The listing builds one solid part. Answer for the finished solid, in the listing's coordinates (mm). A direction names the side the tool comes from. Give positions to 0.01 mm unless a question says otherwise; leave off trailing zeros. Write each loop counter-clockwise with the first axis right and the second up, starting at its lowest first coordinate (ties: lowest second). Pieces come first, ordered by that corner, then holes. Notation, with made-up numbers: (8, 57) -> (60, 57) arc R22 ccw to (60, 71) -> close; hole circle Ø10 at (7.25, -38.5). An arc over 180 degrees is marked (long way). One line per question, with ' | ' between items.
from build123d import *

# Parameters (mm, degrees)
BOSS_EXTRUDE1_DEPTH = 60
FILLET1_R           = 20
FILLET2_R           = 50
SKETCH2_W           = 848.571428571
SKETCH2_H           = 25
CUT_EXTRUDE1_DEPTH  = 1199.832765652
FILLET3_R           = 15
BOSS_EXTRUDE2_DEPTH = 60
CHAMFER1_START      = 59.982172039
CHAMFER1_OUTLINE_W  = 43
CHAMFER1_OUTLINE_H  = 75
CHAMFER1_DEPTH      = 21.017827961
CHAMFER2_START      = 59.982172039
CHAMFER2_OUTLINE_W  = 43
CHAMFER2_OUTLINE_H  = 75
CHAMFER2_DEPTH      = 21.017827961
FILLET4_R           = 5


with BuildPart() as part:
    # Sketch1 → Boss-Extrude1 (new, symmetric)
    with BuildSketch(Plane.XY):
        Polygon((0, 0), (0, -630), (-980, -630), (-980, -645), (-380, -680), (40, -680), (40, 0), align=None)
    extrude(amount=BOSS_EXTRUDE1_DEPTH, both=True)

    # Fillet1
    fillet1_edges = [part.edges().sort_by_distance(p)[0] for p in [
        (0, -630, 0),
    ]]
    fillet(fillet1_edges, radius=FILLET1_R)

    # Fillet2
    fillet2_edges = [part.edges().sort_by_distance(p)[0] for p in [
        (40, -680, 0),
    ]]
    fillet(fillet2_edges, radius=FILLET2_R)

    # Sketch2 → Cut-Extrude1 (cut, through all)
    with BuildSketch(Plane.XY.offset(60)):
        with Locations((-384.285714286, -667.5)):
            Rectangle(SKETCH2_W, SKETCH2_H)
    extrude(amount=-CUT_EXTRUDE1_DEPTH, mode=Mode.SUBTRACT)

    # Fillet3
    fillet3_edges = [part.edges().sort_by_distance(p)[0] for p in [
        (-980, -637.5, 60),
        (-980, -637.5, -60),
    ]]
    fillet(fillet3_edges, radius=FILLET3_R)

    # Sketch4 → Boss-Extrude2 (add, symmetric)
    with BuildSketch(Plane.XY):
        Polygon((40, -45), (80, -45), (80, -112), (62, -112), (55.812506017, -95), (40, -95), align=None)
        Polygon((40, -604), (56.540446486, -604), (62, -589), (80, -589), (80, -599), (70.900744143, -624), (40, -624), align=None)
    extrude(amount=BOSS_EXTRUDE2_DEPTH, both=True)

    # Chamfer1: read off the stored shape, not the designer's step
    # Chamfer1 outline → Chamfer1 (cut)
    with BuildSketch(Plane(origin=(0, 0, 0), x_dir=(0.74035690193716, -0.281696772444383, -0.6103430069628291), z_dir=(0.6722139969935248, 0.3102526139970119, 0.6722139969935248)).offset(CHAMFER1_START)):
        with Locations((33.5, -89.5)):
            Rectangle(CHAMFER1_OUTLINE_W, CHAMFER1_OUTLINE_H)
    extrude(amount=CHAMFER1_DEPTH, mode=Mode.SUBTRACT)

    # Chamfer2: read off the stored shape, not the designer's step
    # Chamfer2 outline → Chamfer2 (cut)
    with BuildSketch(Plane(origin=(0, 0, 0), x_dir=(0.74035690193716, -0.281696772444383, 0.6103430069628291), z_dir=(0.6722139969935248, 0.3102526139970119, -0.6722139969935248)).offset(CHAMFER2_START)):
        with Locations((33.5, 89.5)):
            Rectangle(CHAMFER2_OUTLINE_W, CHAMFER2_OUTLINE_H)
    extrude(amount=CHAMFER2_DEPTH, mode=Mode.SUBTRACT)

    # Fillet4
    # the kernel refuses this fillet: 5 mm, written as the material it adds along each edge
    with BuildSketch(Plane(origin=(40, -624, -60), x_dir=(1, 0, 0), z_dir=(0, 0, 1))) as fillet4_piece_1:
        with BuildLine():
            CenterArc((FILLET4_R, -FILLET4_R), FILLET4_R, 90, 90)
            Line((0, -FILLET4_R), (0, 0))
            Line((0, 0), (FILLET4_R, 0))
        make_face()
    extrude(amount=120)
    # the kernel refuses this fillet: 5 mm, written as the material it takes off along each edge
    with BuildSketch(Plane(origin=(75, -50, 29.869584766), x_dir=(0, 0.45647233632715695, -0.8897376052342775), z_dir=(0.7504731319703868, 0.5880284369504243, 0.30168300503707374))) as fillet4_2_piece_1_section:
        Polygon((-8.486724439, -8.486724439), (8.486724439, -8.486724439), (8.486724439, 8.486724439), (-8.486724439, 8.486724439), align=None)
    fillet4_2_piece_1 = extrude(amount=8.486724439, mode=Mode.PRIVATE)
    fillet4_2_piece_1 = split(fillet4_2_piece_1, bisect_by=Plane(origin=(75, -50, 29.869584766), z_dir=(0, 0.9079593845004515, -0.41905817746174745)), keep=Keep.TOP, mode=Mode.PRIVATE)
    fillet4_2_piece_1 = split(fillet4_2_piece_1, bisect_by=Plane(origin=(75, -50, 29.869584766), z_dir=(0.7071067811865476, 0, -0.7071067811865476)), keep=Keep.TOP, mode=Mode.PRIVATE)
    fillet4_2_piece_1 = split(fillet4_2_piece_1, bisect_by=Plane(origin=(75, -50, 29.869584766), z_dir=(0, 0, 1)), keep=Keep.TOP, mode=Mode.PRIVATE)
    fillet4_2_piece_1 = split(fillet4_2_piece_1, bisect_by=Plane(origin=(80, -50, 29.869584766), z_dir=(-1, 0, 0)), keep=Keep.TOP, mode=Mode.PRIVATE)
    fillet4_2_piece_1 = split(fillet4_2_piece_1, bisect_by=Plane(origin=(78.361069985, -48.44873693, 33.230654751), z_dir=(-0.6722139969935248, -0.3102526139970119, -0.6722139969935248)), keep=Keep.TOP, mode=Mode.PRIVATE)
    fillet4_2_piece_1 = split(fillet4_2_piece_1, bisect_by=Plane(origin=(75, -45, 29.869584766), z_dir=(0, -1, 0)), keep=Keep.TOP, mode=Mode.PRIVATE)
    fillet4_2_piece_1 = fillet4_2_piece_1 - Plane(origin=(75, -50, 29.869584766), x_dir=(-0.7504731319703868, -0.5880284369504243, -0.30168300503707374), z_dir=(0, 0.45647233632715695, -0.8897376052342775)) * Sphere(FILLET4_R, mode=Mode.PRIVATE)
    add(fillet4_2_piece_1, mode=Mode.SUBTRACT)
    with BuildSketch(Plane(origin=(75, -50, -29.869584766), x_dir=(-0.6608271381079537, 0.6608271381079537, -0.3558299974427439), z_dir=(0.7504731319703868, 0.5880284369504243, -0.30168300503707374))) as fillet4_2_piece_2_section:
        Polygon((-8.486724439, -8.486724439), (8.486724439, -8.486724439), (8.486724439, 8.486724439), (-8.486724439, 8.486724439), align=None)
    fillet4_2_piece_2 = extrude(amount=8.486724439, mode=Mode.PRIVATE)
    fillet4_2_piece_2 = split(fillet4_2_piece_2, bisect_by=Plane(origin=(75, -50, -29.869584766), z_dir=(0, 0.9079593845004515, 0.41905817746174745)), keep=Keep.TOP, mode=Mode.PRIVATE)
    fillet4_2_piece_2 = split(fillet4_2_piece_2, bisect_by=Plane(origin=(75, -50, -29.869584766), z_dir=(0, 0, -1)), keep=Keep.TOP, mode=Mode.PRIVATE)
    fillet4_2_piece_2 = split(fillet4_2_piece_2, bisect_by=Plane(origin=(75, -50, -29.869584766), z_dir=(0.7071067811865476, 0, 0.7071067811865476)), keep=Keep.TOP, mode=Mode.PRIVATE)
    fillet4_2_piece_2 = split(fillet4_2_piece_2, bisect_by=Plane(origin=(78.361069985, -48.44873693, -33.230654751), z_dir=(-0.6722139969935248, -0.3102526139970119, 0.6722139969935248)), keep=Keep.TOP, mode=Mode.PRIVATE)
    fillet4_2_piece_2 = split(fillet4_2_piece_2, bisect_by=Plane(origin=(80, -50, -29.869584766), z_dir=(-1, 0, 0)), keep=Keep.TOP, mode=Mode.PRIVATE)
    fillet4_2_piece_2 = split(fillet4_2_piece_2, bisect_by=Plane(origin=(75, -45, -29.869584766), z_dir=(0, -1, 0)), keep=Keep.TOP, mode=Mode.PRIVATE)
    fillet4_2_piece_2 = fillet4_2_piece_2 - Plane(origin=(75, -50, -29.869584766), x_dir=(-0.7504731319703868, -0.5880284369504243, 0.30168300503707374), z_dir=(-0.6608271381079537, 0.6608271381079537, -0.3558299974427439)) * Sphere(FILLET4_R, mode=Mode.PRIVATE)
    add(fillet4_2_piece_2, mode=Mode.SUBTRACT)
    with BuildSketch(Plane(origin=(82.319175466, -115.024880177, 60), x_dir=(-0.9079593845004514, -0.4190581774617474, 0), z_dir=(-0.41905817746174745, 0.9079593845004515, 0))) as fillet4_2_piece_3:
        with BuildLine():
            CenterArc((FILLET4_R * 0.4427405244, -FILLET4_R), FILLET4_R, 90, 47.761827017)
            Line((-FILLET4_R * 0.297616377538, -FILLET4_R * 0.327786003006), (0, 0))
            Line((0, 0), (FILLET4_R * 0.4427405244, 0))
        make_face()
    extrude(amount=82.657618428, mode=Mode.SUBTRACT)
    with BuildSketch(Plane(origin=(80, -45, 29.869584766), x_dir=(-1, 0, 0), z_dir=(0, 0, -1))) as fillet4_2_piece_4:
        with BuildLine():
            CenterArc((FILLET4_R, -FILLET4_R), FILLET4_R, 90, 90)
            Line((0, -FILLET4_R), (0, 0))
            Line((0, 0), (FILLET4_R, 0))
        make_face()
    extrude(amount=59.739169533, mode=Mode.SUBTRACT)
    with BuildSketch(Plane(origin=(80, -115.024880177, 62.319175466), x_dir=(0, -0.41905817746174745, -0.9079593845004515), z_dir=(0, 0.9079593845004515, -0.41905817746174745))) as fillet4_2_piece_5:
        with BuildLine():
            CenterArc((FILLET4_R * 0.4427405244, FILLET4_R), FILLET4_R, 222.238172983, 47.761827017)
            Line((-FILLET4_R * 0.297616377538, FILLET4_R * 0.327786003006), (0, 0))
            Line((0, 0), (FILLET4_R * 0.4427405244, 0))
        make_face()
    extrude(amount=72.63821652, mode=Mode.SUBTRACT)
    with BuildSketch(Plane(origin=(77.565207617, -45, 32.434792383), x_dir=(-0.7071067811865476, 0, -0.7071067811865476), z_dir=(-0.7071067811865476, 0, 0.7071067811865476)), Plane(origin=(43.586980958, -45, -66.413019041), x_dir=(-0.7071067811865476, 0, 0.7071067811865476), z_dir=(0.7071067811865476, 0, 0.7071067811865476))) as fillet4_2_piece_6:
        with BuildLine():
            CenterArc((FILLET4_R * 0.725550280312, FILLET4_R), FILLET4_R, 198.074454838, 71.925545162)
            Line((-FILLET4_R * 0.225103871053, FILLET4_R * 0.689747386003), (0, 0))
            Line((0, 0), (FILLET4_R * 0.725550280312, 0))
        make_face()
    extrude(amount=48.052468966, mode=Mode.SUBTRACT)
    with BuildSketch(Plane(origin=(80, -49.072329814, -31.879536837), x_dir=(-0.7403569019371568, 0.2816967724443845, -0.6103430069628323), z_dir=(0, -0.9079593845004515, -0.41905817746174745))) as fillet4_2_piece_7:
        with BuildLine():
            CenterArc((FILLET4_R * 0.4427405244, -FILLET4_R), FILLET4_R, 90, 47.761827017)
            Line((-FILLET4_R * 0.297616377538, -FILLET4_R * 0.327786003006), (0, 0))
            Line((0, 0), (FILLET4_R * 0.4427405244, 0))
        make_face()
    extrude(amount=72.63821652, mode=Mode.SUBTRACT)
    with BuildSketch(Plane(origin=(82.319175466, -115.024880177, -60), x_dir=(-0.9079593845004514, -0.4190581774617474, 0), z_dir=(-0.41905817746174745, 0.9079593845004515, 0))) as fillet4_2_piece_8:
        with BuildLine():
            CenterArc((FILLET4_R * 0.4427405244, FILLET4_R), FILLET4_R, 222.238172983, 47.761827017)
            Line((-FILLET4_R * 0.297616377538, FILLET4_R * 0.327786003006), (0, 0))
            Line((0, 0), (FILLET4_R * 0.4427405244, 0))
        make_face()
    extrude(amount=82.657618428, mode=Mode.SUBTRACT)
    with BuildSketch(Plane(origin=(80, -112, 72.5), x_dir=(0, 1, 0), z_dir=(0, 0, -1)), Plane(origin=(80, -589, 72.5), x_dir=(-1, 0, 0), z_dir=(0, 0, -1))) as fillet4_2_piece_9:
        with BuildLine():
            CenterArc((FILLET4_R, -FILLET4_R), FILLET4_R, 90, 90)
            Line((0, -FILLET4_R), (0, 0))
            Line((0, 0), (FILLET4_R, 0))
        make_face()
    extrude(amount=145, mode=Mode.SUBTRACT)
    with BuildSketch(Plane(origin=(70.900744143, -624, -68.752594228), x_dir=(0.34202014332566244, 0.9396926207859106, 0), z_dir=(0, 0, 1))) as fillet4_2_piece_10:
        with BuildLine():
            CenterArc((FILLET4_R * 0.70020753821, FILLET4_R), FILLET4_R, 200, 70)
            Line((-FILLET4_R * 0.239485082576, FILLET4_R * 0.657979856674), (0, 0))
            Line((0, 0), (FILLET4_R * 0.70020753821, 0))
        make_face()
    extrude(amount=137.505188455, mode=Mode.SUBTRACT)
    with BuildSketch(Plane(origin=(80, -599, 62.204087259), x_dir=(0, 1, 0), z_dir=(0, 0, -1))) as fillet4_2_piece_11:
        with BuildLine():
            CenterArc((FILLET4_R * 0.176326980708, -FILLET4_R), FILLET4_R, 90, 20)
            Line((-FILLET4_R * 0.165693162617, -FILLET4_R * 0.0603073792141), (0, 0))
            Line((0, 0), (FILLET4_R * 0.176326980708, 0))
        make_face()
    extrude(amount=124.408174518, mode=Mode.SUBTRACT)


solid = part.part
Item 1: Consider line 1 (X direction, y = -368.5, z = 6); line 2 (Y direction, x = -713, z = -42.5); line 3 (X direction, y = -591, z = -10). Determine where each line is inside the solid, lowest interval first. Write a range as [from, to].
Answers below:
line 1: [0, 40] | line 2: [-655, -630] | line 3: [0, 40], [61.27, 79]
Item 2: Flat-ended cylindrical pins translate along their axes: pin 1 (8 mm diameter, centred on x = 51, z = 28, fed in from -Y); pin 2 (10.5 mm diameter, centred on x = 70, z = 26, fed in from +Y); pin 3 (10 mm diameter, centred on x = -489, z = 41.5, fed in from +Y). Find the tip coordinate at first contact, or state that the pin passes through.
Answers below:
pin 1: y = -624 | pin 2: y = -45 | pin 3: y = -630
Item 3: A tool of negligible diameter and unlimited length cuts with its end or side. For faces 1 (the face through (56, -624, 1)), 2 (the face through (64.96, -77.81, -59.56)), 3 (the face through (-493, -630, 1)), 4 (the face through (-394, -655, 1)), 5 (the face through (40, -23, 1)), from which of +Z, -Z, +X, -X, +Y, -Y can it reach the whole face along a straight path? Write none if from no direction.
Answers below:
face 1: +Z, -Z, +X, -Y | face 2: -Z, +X, +Y | face 3: +Z, -Z, -X, +Y | face 4: +Z, -Z, +X, -X, -Y | face 5: +Z, -Z, +X, +Y
Item 4: Determine the mould class of faces 6 (the face through (40, -353, 1)), 7 (the face through (61.825, -45.979, -47.247)), 8 (the face through (-208, -641, -60)) for opening direction Y: pulls with the +Y half, pulls with the -Y half, needs draft (parallel to the pull), parting line crosses it, or undercut.
Answers below:
face 6: undercut | face 7: pulls with the +Y half | face 8: needs draft
Item 5: Find section A-A (z = -14.5). Write down the section's boundary in (x, y).
Answers below:
outline: (-980, -645) -> (-808.57, -655) -> (33.3, -655) arc R50 ccw to (40, -630) -> (40, -629) arc R5 cw to (45, -624) -> (67.4, -624) arc R5 ccw to (72.1, -620.71) -> (79.7, -599.83) arc R5 ccw to (80, -598.12) -> (80, -594) arc R5 ccw to (75, -589) -> (62, -589) -> (56.54, -604) -> (40, -604) -> (40, -95) -> (55.81, -95) -> (62, -112) -> (75, -112) arc R5 ccw to (80, -107) -> (80, -50) arc R5 ccw to (75, -45) -> (40, -45) -> (40, 0) -> (0, 0) -> (0, -610) arc R20 cw to (-20, -630) -> (-980, -630) -> close
Item 6: Find section B-B (y = -218). Write down the section's boundary in (x, z).
Answers below:
outline: (0, -60) -> (40, -60) -> (40, 60) -> (0, 60) -> close
Item 7: Find section C-C (x = -146). Write down the section's boundary in (y, z), then the cut area to 3 significant figures.
Answers below:
outline: (-655, -60) -> (-630, -60) -> (-630, 60) -> (-655, 60) -> close | area: 3,000 mm²
